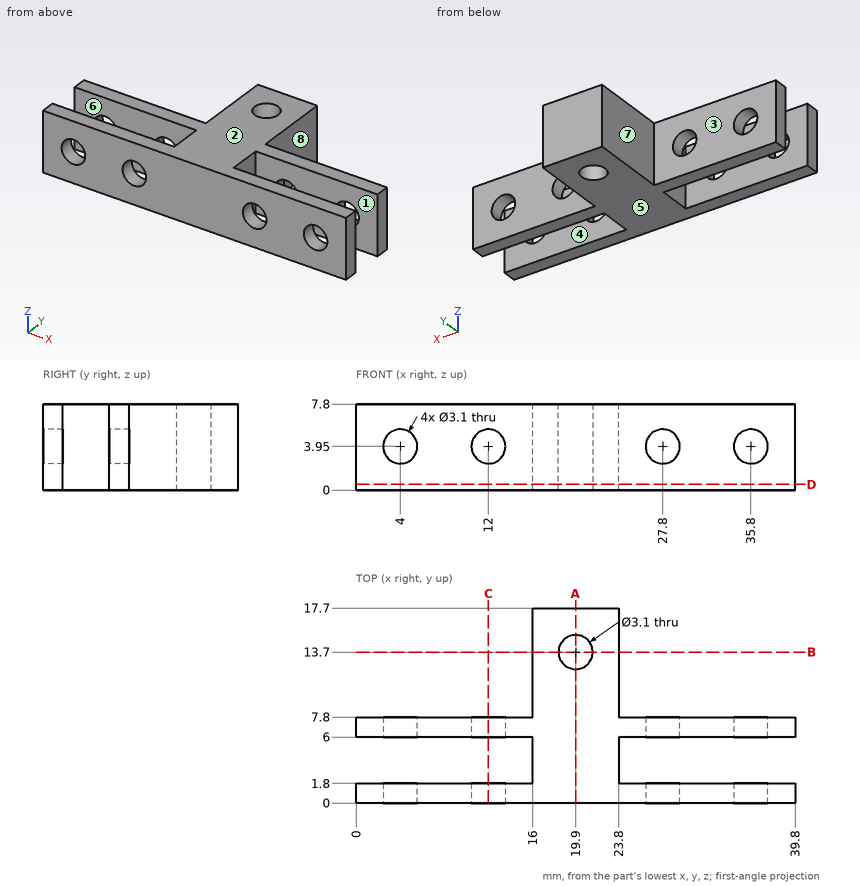
Geometry: see drawing. Coordinates: mm, zero at the bounding-box minimum. A direction names the side the tool comes from. Give positions to 0.01 mm unless a question says otherwise; leave off trailing zeros. Loops run counter-clockwise (first coordinate to the right, second up) from the corner with the lowest first, then second, coordinate; pieces in that order, holes last. Notation, with made-up numbers: (6.25, -12.75) -> (51.25, -12.75) arc R20 ccw to (51.25, 7.25) -> close; hole circle Ø7 at (20.5, 72). An arc over 180 degrees is marked (long way). Use one line per item in the form item = value.
Item 1: Section query A-A on x = 19.9. Output: boundary loops of the cut face in (y, z), and give its area (3 significant figures).
A:
outline = (0, 0) -> (12.15, 0) -> (12.15, 7.8) -> (0, 7.8) -> close; (15.25, 0) -> (17.7, 0) -> (17.7, 7.8) -> (15.25, 7.8) -> close
area = 114 mm^2
Item 2: Line query: probe 1 along Y at (x, z) = (30, 1.25); probe 2 along Z at (x, y) = (35.8, 0.4); probe 3 along X at (y, z) = (5.5, 3). Output: solid intervals per line, ascending.
A:
probe_1 = 0 to 1.8, 6 to 7.8
probe_2 = 0 to 2.4, 5.5 to 7.8
probe_3 = 16 to 23.8
Item 3: Pin query (flat end, axial travel): P1, Ø2.5, axis at y = 14, z = 4.5, coming from the -X side; P2, Ø3, axis at y = 14.5, z = 4.5, coming from the +X side; P3, Ø3.5, axis at x = 4, z = 3.95, coming from the +Y side. Return the tip coordinate at first contact, or that it passes through.
A:
P1 = 16
P2 = 23.8
P3 = 7.8
Item 4: Section query D-D on z = 0.5. Output: boundary loops of the cut face in (x, y), and give its area (3 significant figures).
A:
outline = (0, 0) -> (39.8, 0) -> (39.8, 1.8) -> (23.8, 1.8) -> (23.8, 6) -> (39.8, 6) -> (39.8, 7.8) -> (23.8, 7.8) -> (23.8, 17.7) -> (16, 17.7) -> (16, 7.8) -> (0, 7.8) -> (0, 6) -> (16, 6) -> (16, 1.8) -> (0, 1.8) -> close; hole circle Ø3.1 at (19.9, 13.7)
area = 246 mm^2
Item 5: Access query for the marked faces 4, 5, 6, 7 and 8. Directions: +Z, -Z, +X, -X, +Y, -Y. A direction counts if a zero-diameter tool reaches every point of the face in a straight line with its end or side. Return the directions, or none.
A:
face_4 = +Z, -Z, +X
face_5 = -Z, +X, -X, +Y, -Y
face_6 = +Z, -Z, -X
face_7 = +Z, -Z, -X, +Y
face_8 = +Z, -Z, +X, +Y
Item 6: Section query C-C on x = 12. Output: boundary loops of the cut face in (y, z), and give its area (3 significant figures).
A:
outline = (0, 0) -> (1.8, 0) -> (1.8, 2.4) -> (0, 2.4) -> close; (0, 5.5) -> (1.8, 5.5) -> (1.8, 7.8) -> (0, 7.8) -> close; (6, 0) -> (7.8, 0) -> (7.8, 2.4) -> (6, 2.4) -> close; (6, 5.5) -> (7.8, 5.5) -> (7.8, 7.8) -> (6, 7.8) -> close
area = 16.9 mm^2
Item 7: Draft query along Y for the marked faces 1, 2 and 3. Return one class per face: pulls with the +Y half, pulls with the -Y half, needs draft (parallel to the pull), parting line crosses it, or undercut.
A:
face_1 = undercut
face_2 = needs draft
face_3 = pulls with the +Y half
Item 8: Section query B-B on y = 13.7. Output: boundary loops of the cut face in (x, z), and give its area (3 significant figures).
A:
outline = (16, 0) -> (18.35, 0) -> (18.35, 7.8) -> (16, 7.8) -> close; (21.45, 0) -> (23.8, 0) -> (23.8, 7.8) -> (21.45, 7.8) -> close
area = 36.7 mm^2
